Model file for the job. Use its own axes, mm. A direction names the side the tool comes from. Coordinates: 2 decimals unless noted, no trailing zeros. Order: outer loops, then holes, each group sorted by start corner. A loop starts at its lowest first (then second) coordinate and runs counter-clockwise, first axis right, second up.
from build123d import *

# Parameters (mm, degrees)
SKETCH1_R           = 7.25
BOSS_EXTRUDE1_DEPTH = 16.5
FILLET1_R           = 1
SKETCH4_R           = 3
BOSS_EXTRUDE2_DEPTH = 1
SKETCH5_R           = 0.295
CUT_EXTRUDE2_DEPTH  = 10


with BuildPart() as part:
    # Sketch1 → Boss-Extrude1 (new body)
    with BuildSketch(Plane(origin=(0, 0, 0), x_dir=(1, 0, 0), z_dir=(0, 1, 0))):
        with Locations(Location((0, 0, 0), (0, 0, 270))):
            Circle(SKETCH1_R)
    extrude(amount=BOSS_EXTRUDE1_DEPTH)

    # Fillet1
    fillet1_edges = [part.edges().sort_by_distance(p)[0] for p in [
        (0, 16.5, -7.25),
    ]]
    fillet(fillet1_edges, radius=FILLET1_R)

    # Sketch4 → Boss-Extrude2 (add)
    with BuildSketch(Plane.XZ):
        with Locations(Location((0, 0, 0), (0, 0, 90))):
            Circle(SKETCH4_R)
    extrude(amount=BOSS_EXTRUDE2_DEPTH)

    # Sketch5 → Cut-Extrude2 (cut)
    with BuildSketch(Plane.XZ.offset(1)):
        with Locations(Location((0, 0, 0), (0, 0, 270))):
            Circle(SKETCH5_R)
    extrude(amount=-CUT_EXTRUDE2_DEPTH, mode=Mode.SUBTRACT)


solid = part.part
Q1. Which spindle directions (+Z, -Z, +X, -X, +Y, -Y) get a long thin tool onto all of the face, cutting with end or side? Do faces 1 (the face through (-0.9, -0.49, 2.86)), 2 (the face through (-2.777, 7.642, 6.697)). Say none if no direction does.
Established:
face 1: -Y
face 2: +Y, -Y
Q2. Cut at A-A, the plane z = 0. List the corners of the cut face in (x, y) (3 decimals).
Established:
outline: (-7.25, 0) - (-3, 0) - (-3, -1) - (-0.295, -1) - (-0.295, 9) - (0.295, 9) - (0.295, -1) - (3, -1) - (3, 0) - (7.25, 0) - (7.25, 15.5) arc R1 ccw to (6.25, 16.5) - (-6.25, 16.5) arc R1 ccw to (-7.25, 15.5) - close
Q3. Cut at B-B, the plane x = 0. List the corners of the cut face in (y, z) (3 decimals).
Established:
outline: (-1, -3) - (0, -3) - (0, -7.25) - (15.5, -7.25) arc R1 ccw to (16.5, -6.25) - (16.5, 6.25) arc R1 ccw to (15.5, 7.25) - (0, 7.25) - (0, 3) - (-1, 3) - (-1, 0.295) - (9, 0.295) - (9, -0.295) - (-1, -0.295) - close
Q4. Cut at C-C, the plane y = 12.25. List the corners of the cut face in (x, z), plus the area to 3 significant figures.
Established:
outline: circle Ø14.5 at (0, 0)
area: 165 mm2
Q5. Drop flat-ended pins along their axis: P1, Ø1, axis at x = 1, y = 13, coming from the -Z side; P2, Ø1.5, axis at x = -4.5, y = 14, coming from the +Z side; P3, Ø1, axis at y = 7.5, z = -1, coming from the -X side. Give the stop position or say it passes through.
Established:
P1: stops at z = -7.23
P2: stops at z = 6.2
P3: stops at x = -7.23
Q6. Probe line 1 (X direction, y = 3.25, z = 0) (3 decimals); line 2 (Y direction, x = 3, z = 4); line 3 (Y direction, x = -4.75, z = -5). List the from-to ranges inside material, lowest first.
Established:
line 1: x = -7.25 to -0.295, 0.295 to 7.25
line 2: y = 0 to 16.5
line 3: y = 0 to 16.26
